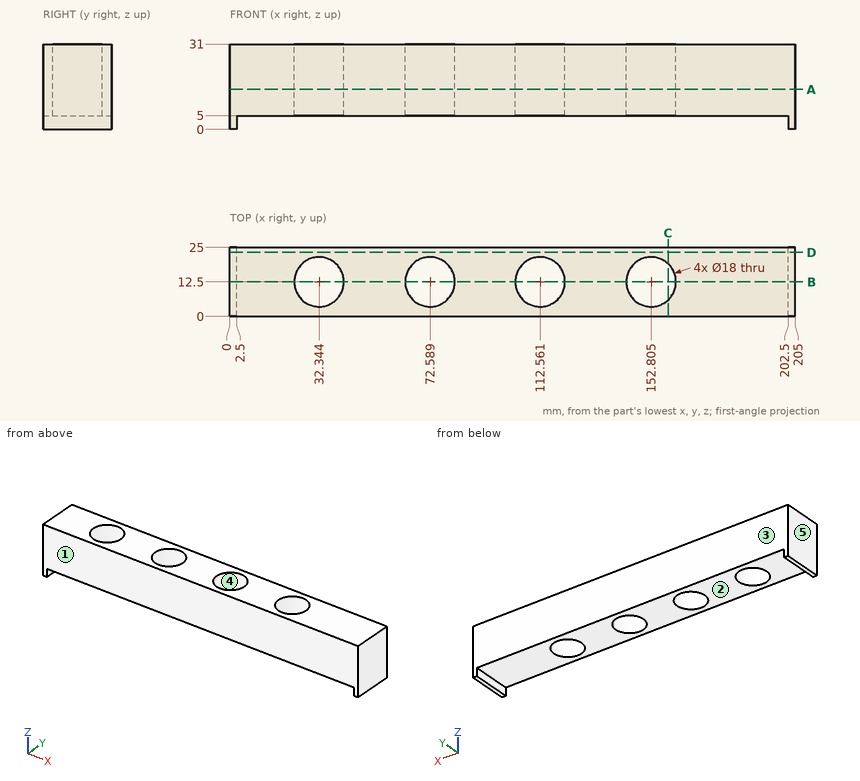
Could you check a few things on this drawing? It's one solid part, dimensions in mm from its lowest x, y, z. A direction names the side the tool comes from. Give positions to 0.01 mm unless a question says otherwise; leave off trailing zeros. Order: outer loops, then holes, each group sorted by start corner. A loop starts at its lowest first (then second) coordinate and runs counter-clockwise, first axis right, second up. Notation, with made-up numbers: (23, 35.25) - (80, 35.25) arc R29 ccw to (80, 69.25) - close; hole circle Ø1 at (-32.5, 68.25). An arc over 180 degrees is marked (long way). Answer as a JSON object with one key per item and string values. Group by question number.
Item 1: For P1, Ø3, axis at y = 21, z = 24.5, coming from the -X side; P2, Ø6, axis at x = 85, y = 6.5, coming from the -Z side; P3, Ø3, axis at x = 36.5, y = 8, coming from the +Z side, each with a flat end and sliding along its axis, tell me the tip position at first contact or that it passes through.
Item 2: Which directions (+Z, -Z, +X, -X, +Y, -Y) give clear straight access to the entire face, cutting with the end or side of a thin tool? Please do the marked faces 1 and 2.
Item 3: Please list where these lines run through material, in increasing order: probe 1 along X at (y, z) = (13, 29) (1 decimal); probe 2 along X at (y, z) = (9.5, 12.5) (1 decimal); probe 3 along Z at (x, y) = (48.5, 20.5).
Item 4: If we section it at B-B on y = 12.5: Please give me the cut outline in (x, z) (1 decimal).
Item 5: If we section it at A-A on z = 14.5: Please give me the cut outline in (x, y) (1 decimal).
Item 6: If we section it at D-D on y = 23.25: Please give me the cut outline in (x, z), and give its area (4 significant figures).
Item 7: If we section it at C-C on x = 159: Please give me the cut outline in (y, z).
Item 8: If we mould it in two halves opening along Y, with no side actions, what happens to the marked faces 3, 4 and 5? For each: pulls with the +Y half, pulls with the -Y half, needs draft (parallel to the pull), parting line crosses it, or undercut.
Result set:
{
 "1": {"P1": "x = 0", "P2": "z = 5", "P3": "through"},
 "2": {"face 1": "+Z, -Z, +X, -X, -Y", "face 2": "-Z, +Y, -Y"},
 "3": {"probe 1": "0 to 23.4, 41.3 to 63.6, 81.6 to 103.6, 121.5 to 143.8, 161.8 to 205", "probe 2": "0 to 23.9, 40.8 to 64.1, 81.1 to 104.1, 121 to 144.3, 161.3 to 205", "probe 3": "5 to 31"},
 "4": {"outline": "(0, 0) - (2.5, 0) - (2.5, 5) - (23.3, 5) - (23.3, 31) - (0, 31) - close; (41.3, 5) - (63.6, 5) - (63.6, 31) - (41.3, 31) - close; (81.6, 5) - (103.6, 5) - (103.6, 31) - (81.6, 31) - close; (121.6, 5) - (143.8, 5) - (143.8, 31) - (121.6, 31) - close; (161.8, 5) - (202.5, 5) - (202.5, 0) - (205, 0) - (205, 31) - (161.8, 31) - close"},
 "5": {"outline": "(0, 0) - (205, 0) - (205, 25) - (0, 25) - close; hole circle Ø18 at (32.3, 12.5); hole circle Ø18 at (72.6, 12.5); hole circle Ø18 at (112.6, 12.5); hole circle Ø18 at (152.8, 12.5)"},
 "6": {"outline": "(0, 0) - (2.5, 0) - (2.5, 5) - (202.5, 5) - (202.5, 0) - (205, 0) - (205, 31) - (0, 31) - close", "area": "5,355 mm²"},
 "7": {"outline": "(0, 5) - (5.97, 5) - (5.97, 31) - (0, 31) - close; (19.03, 5) - (25, 5) - (25, 31) - (19.03, 31) - close"},
 "8": {"face 3": "pulls with the +Y half", "face 4": "undercut", "face 5": "needs draft"}
}
